Source: CAD feature listing. Evaluate the final solid. Frame: model axes, mm. Round coordinates to 2 decimals unless told otherwise and drop trailing zeros. Write each loop counter-clockwise with the first axis right and the second up, starting at its lowest first coordinate (ties: lowest second). Pieces come first, ordered by that corner, then holes.
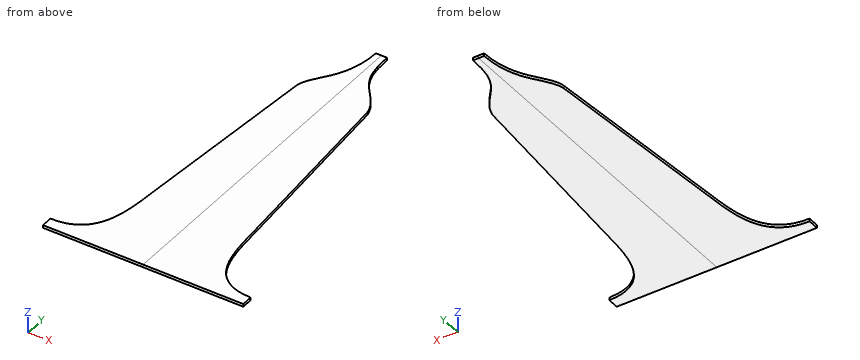
Autodesk Inventor part; units mm, degrees
ref_plane "YZ Plane" through (0, 0, 0) normal (1, 0, 0) x (0, 1, 0)
ref_plane "XZ Plane" through (0, 0, 0) normal (0, 1, 0) x (-1, 0, 0)
ref_plane "XY Plane" through (0, 0, 0) normal (0, 0, 1) x (1, 0, 0)
sketch "Sketch1" plane through (0, 0, 0) normal (0, 0, 1) x (1, 0, 0)
  line L0 (76.2, -12.7) -> (381, -12.7) construction
  line L1 (-76.2, -12.7) -> (-381, -12.7) construction
  line L2 (-76.2, 0) -> (-381, 0) construction
  line L3 (76.2, 0) -> (381, 0) construction
  line L4 (0, -116.2267) -> (0, 608.4603)
  line L5 (0, -12.7) -> (-114.6099, -12.7)
  line L6 (-114.6099, -12.7) -> (-114.6099, 0)
  line L7 (0, 394.3626) -> (-6.35, 394.3626)
  line L8 (-40.2136, 308.3016) -> (-57.305, 93.11)
  spline S0 degree 3 poles (-114.6099, 0) (-60.3377, 0) (-60.3484, 54.7909) (-57.305, 93.11) knots 0 0 0 0 1 1 1 1
  line L9 (-119.6474, 0) -> (-109.5725, 0) construction
  arc A0 (-118.6349, 0.1005) -> (-110.585, 0.1005) centre (-114.6099, 80.6377) ccw construction
  line L10 (40.2136, 308.3016) -> (57.305, 93.11)
  line L11 (0, 394.3626) -> (6.35, 394.3626)
  spline S1 degree 3 poles (114.6099, 0) (60.3377, 0) (60.3484, 54.7909) (57.305, 93.11) knots 0 0 0 0 1 1 1 1
  line L12 (119.6474, 0) -> (109.5725, 0) construction
  arc A1 (110.585, 0.1005) -> (118.6349, 0.1005) centre (114.6099, 80.6377) ccw construction
  line L13 (0, -12.7) -> (114.6099, -12.7)
  line L14 (114.6099, -12.7) -> (114.6099, 0)
  spline S2 degree 4 poles (-6.35, 394.3626) (-6.35, 372.6715) (-17.579, 345.2739) (-20.8089, 340.9314) (-39.3875, 318.7028) (-40.2136, 308.3016) knots 0 0 0 0 0 0.523271 1 1 1 1 1
  line L15 (-6.35, 421.2444) -> (-6.35, 367.4808) construction
  arc A2 (-8.4521, 373.2806) -> (-8.4521, 415.4446) centre (-113.1163, 394.3626) ccw construction
  spline S3 degree 4 poles (6.35, 394.3626) (6.35, 352.9097) (13.7895, 346.0085) (38.4808, 330.1195) (40.2136, 308.3016) knots 0 0 0 0 0 1 1 1 1 1
  line L16 (6.35, 421.2444) -> (6.35, 367.4808) construction
  arc A3 (8.4521, 415.4446) -> (8.4521, 373.2806) centre (113.1163, 394.3626) ccw construction
  line L17 (-14.8603, 351.5845) -> (-28.3954, 331.1958) construction
  arc A4 (-27.429, 333.5531) -> (-16.6575, 349.7787) centre (-101.0508, 394.1155) ccw construction
  point P0 (0, 0)
  point P1 (-21.6278, 341.3901)
  point P2 (21.6278, 341.3901)
  dimension "d0" = 6.35
extrude "Extrusion1" add sketch "Sketch1" against normal blind 3.175
properties part number "Bottom Plate v1" material "Wood (Cherry)"
Q1. Line query: line 1 (X direction, y = 292.5, z = -1.8); line 2 (Y direction, x = -98, z = -3); line 3 (X direction, y = 252.5, z = -1.7). Output: solid intervals per line, ascending.
Q2. Section query B-B, the plane x = -45. Output: boundary loops of the cut face in (y, z) (3 decimals).
Q3. Section query A-A, the plane y = 219. Output: boundary loops of the cut face in (x, z) (3 decimals).
Q4. Pin query (flat end, axial travel): P1, Ø1, axis at y = 147, z = -1.5, coming from the +X side. Return the tip coordinate at first contact, or that it passes through.
Filled in:
1. line 1: x = -41.47 to 41.47
1. line 2: y = -12.7 to 2.05
1. line 3: x = -44.65 to 44.65
2. outline: (-12.7, -3.175) - (248.038, -3.175) - (248.038, 0) - (-12.7, 0) - close
3. outline: (-47.306, -3.175) - (47.306, -3.175) - (47.306, 0) - (-47.306, 0) - close
4. P1: stops at x = 53.06
